from build123d import *

# Parameters (mm, degrees)
SKETCH1_W                                      = 60.6552
SKETCH1_H                                      = 128.4986
BOSS_EXTRUDE1_DEPTH                            = 2.54
CSK_FOR_M3_FLAT_HEAD_MACHINE_SCREW1_AT_2_COUNT = 2
CSK_FOR_M3_FLAT_HEAD_MACHINE_SCREW1_AT_2_PITCH = 75.0062
M3_CLEARANCE_SLOT1_DEPTH                       = 2.54
F_1_4_CLEARANCE_HOLE1_D                        = 7.14248
F_1_4_CLEARANCE_HOLE2_D                        = 6.5278
F_3_8_CLEARANCE_HOLE2_D                        = 10.0838
F_10_CLEARANCE_HOLE1_D                         = 5.6134
CSK_FOR_M2_5_FLAT_HEAD_MACHINE_SCREW1_AT_COUNT = 2
CSK_FOR_M2_5_FLAT_HEAD_MACHINE_SCREW1_AT_PITCH = 25.4
F_11_64_0_17188_DIAMETER_HOLE1_D               = 4.365752
F_6_CLEARANCE_HOLE1_D                          = 4.3053


# Read off the part's stored shape, not the designer's step: M3 Clearance Slot1
with BuildPart() as part:
    # Sketch1 → Boss-Extrude1 (new body)
    with BuildSketch(Plane(origin=(0, 0, 0), x_dir=(1, 0, 0), z_dir=(0, 1, 0))):
        Rectangle(SKETCH1_W, SKETCH1_H)
    extrude(amount=BOSS_EXTRUDE1_DEPTH)

    # Sketch5 → CSK for M3 Flat Head Machine Screw1 (revolve, cut)
    with BuildSketch(Plane(origin=(25.4, 0, -37.5031), x_dir=(0, 0, -1), z_dir=(1, 0, 0))):
        Polygon((0, 0), (0, 2.54), (1.8, 2.54), (1.8, 1.35), (3.15, 0), align=None)
    csk_for_m3_flat_head_machine_screw1 = revolve(axis=Axis((25.4, -6.35, -37.5031), (0, 1, 0)), mode=Mode.SUBTRACT)

    # CSK for M3 Flat Head Machine Screw1 at 2: CSK for M3 Flat Head Machine Screw1 ×2
    with Locations(*[(0, 0, i * CSK_FOR_M3_FLAT_HEAD_MACHINE_SCREW1_AT_2_PITCH) for i in range(1, CSK_FOR_M3_FLAT_HEAD_MACHINE_SCREW1_AT_2_COUNT)]):
        add(csk_for_m3_flat_head_machine_screw1, mode=Mode.SUBTRACT)

    # M3 Clearance Slot1 outline → M3 Clearance Slot1 (cut)
    with BuildSketch(Plane(origin=(0, 0, 0), x_dir=(1, 0, 0), z_dir=(0, 1, 0))):
        with BuildLine():
            ThreePointArc((24.11, -63.0021), (25.86, -61.2521), (24.11, -59.5021))
            Line((24.11, -59.5021), (21.61, -59.5021))
            ThreePointArc((21.61, -59.5021), (19.86, -61.2521), (21.61, -63.0021))
            Line((21.61, -63.0021), (24.11, -63.0021))
        make_face()
        with BuildLine():
            ThreePointArc((24.11, 59.5021), (25.86, 61.2521), (24.11, 63.0021))
            Line((24.11, 63.0021), (21.61, 63.0021))
            ThreePointArc((21.61, 63.0021), (19.86, 61.2521), (21.61, 59.5021))
            Line((21.61, 59.5021), (24.11, 59.5021))
        make_face()
    m3_clearance_slot1 = extrude(amount=M3_CLEARANCE_SLOT1_DEPTH, mode=Mode.SUBTRACT)

    # Mirror1: CSK for M3 Flat Head Machine Screw1, M3 Clearance Slot1 across plane
    add(csk_for_m3_flat_head_machine_screw1.mirror(Plane(origin=(0, 0, 0), x_dir=(0, 0, 1), z_dir=(1, 0, 0))), mode=Mode.SUBTRACT)
    add(m3_clearance_slot1.mirror(Plane(origin=(0, 0, 0), x_dir=(0, 0, 1), z_dir=(1, 0, 0))), mode=Mode.SUBTRACT)

    # Mirror1 copy 1 sketch → Mirror1 copy 1 (revolve, cut)
    with BuildSketch(Plane(origin=(-25.4, 0, 37.5031), x_dir=(0, 0, -1), z_dir=(-1, 0, 0))):
        Polygon((0, 0), (0, -2.54), (1.8, -2.54), (1.8, -1.35), (3.15, 0), align=None)
    revolve(axis=Axis((-25.4, -6.35, 37.5031), (0, -1, 0)), mode=Mode.SUBTRACT)

    # 1/4 Clearance Hole1 (through all)
    with Locations(Plane(origin=(0, 0, 0), x_dir=(-1, 0, 0), z_dir=(0, -1, 0))):
        with Locations((16.3576, 35.0012), (16.3576, 21.301199968), (16.3576, -32.798800036)):
            Hole(F_1_4_CLEARANCE_HOLE1_D / 2)

    # 1/4 Clearance Hole2 (through all)
    with Locations(Plane(origin=(0, 0, 0), x_dir=(-1, 0, 0), z_dir=(0, -1, 0))):
        with Locations((-12.2174, 35.0012), (2.0701, 35.0012), (2.0701, 21.301199968), (-12.2174, 21.301199968), (-12.2174, -17.08879996), (2.0701, -32.798800036)):
            Hole(F_1_4_CLEARANCE_HOLE2_D / 2)

    # 3/8 Clearance Hole2 (through all)
    with Locations(Plane(origin=(0, 0, 0), x_dir=(-1, 0, 0), z_dir=(0, -1, 0))):
        with Locations((9.7536, -17.08879996), (-5.07365, 2.731200024)):
            Hole(F_3_8_CLEARANCE_HOLE2_D / 2)

    # #10 Clearance Hole1 (through all)
    with Locations(Plane(origin=(0, 0, 0), x_dir=(-1, 0, 0), z_dir=(0, -1, 0))):
        with Locations((-12.2174, -32.798800036)):
            Hole(F_10_CLEARANCE_HOLE1_D / 2)

    # Sketch73 → CSK for M2.5 Flat Head Machine Screw1 (revolve, cut)
    with BuildSketch(Plane(origin=(-12.7, 2.54, 49.2633), x_dir=(0, 0, 1), z_dir=(1, 0, 0))):
        Polygon((0, 0), (0, 2.54), (1.45, 2.54), (1.45, 1.3), (2.75, 0), align=None)
    csk_for_m2_5_flat_head_machine_screw1 = revolve(axis=Axis((-12.7, 8.89, 49.2633), (0, -1, 0)), mode=Mode.SUBTRACT)

    # CSK for M2.5 Flat Head Machine Screw1 at: CSK for M2.5 Flat Head Machine Screw1 ×2
    with Locations(*[(i * CSK_FOR_M2_5_FLAT_HEAD_MACHINE_SCREW1_AT_PITCH, 0, 0) for i in range(1, CSK_FOR_M2_5_FLAT_HEAD_MACHINE_SCREW1_AT_COUNT)]):
        add(csk_for_m2_5_flat_head_machine_screw1, mode=Mode.SUBTRACT)

    # 11/64 (0.17188) Diameter Hole1 (through all)
    with Locations(Plane(origin=(0, 0, 0), x_dir=(-1, 0, 0), z_dir=(0, -1, 0))):
        with Locations((11.938, 9.731199994), (11.938, 2.731200024), (11.938, -4.268799946)):
            Hole(F_11_64_0_17188_DIAMETER_HOLE1_D / 2)

    # #6 Clearance Hole1 (through all)
    with Locations(Plane(origin=(0, 2.54, 0), x_dir=(1, 0, 0), z_dir=(0, 1, 0))):
        with Locations((-22.567944323, 48.012104001), (-22.567944323, -48.012104001)):
            f_6_clearance_hole1 = Hole(F_6_CLEARANCE_HOLE1_D / 2)

    # Mirror2: #6 Clearance Hole1 across plane
    add(f_6_clearance_hole1.mirror(Plane(origin=(0, 0, 0), x_dir=(0, 0, 1), z_dir=(1, 0, 0))), mode=Mode.SUBTRACT)


solid = part.part
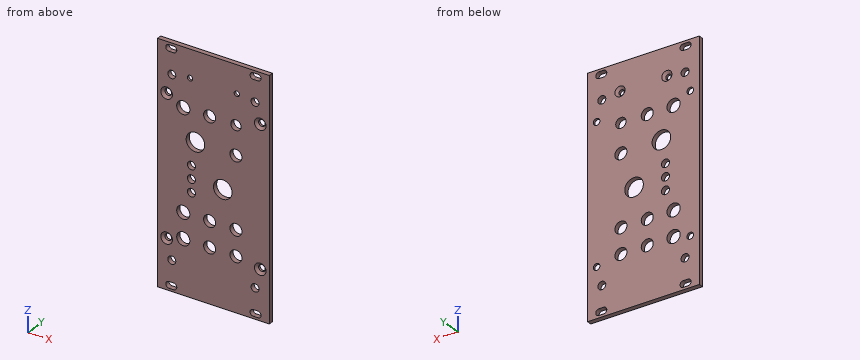
Geometry check sheet. Reference: the model listing, model coordinates, mm. Round coordinates to 2 decimals unless told otherwise and drop trailing zeros. Order: outer loops, then holes, each group sorted by start corner. A loop starts at its lowest first (then second) coordinate and runs counter-clockwise, first axis right, second up. Notation, with made-up numbers: M -32.5,-39.5 L 10.5,-39.5 A21 ccw 10.5,-9.5 Z; hole C 76.25,-2 d9. An arc over 180 degrees is marked long. Answer in a Markdown table with one row per item. Add a question column.
Item 1: Sectioned sample at B-B, the plane z = -20. Enter the section's corners in (x, y).
Item 2: Sectioned sample at A-A, the plane x = 12.7. Enter the section's corners in (y, z), plus the area to 3 significant figures.
Item 3: Depth check by flat-ended pin: pin 1 Ø2.5 at (x, z) = (22.57, 48.01) entering from +Y. Enter the tip coordinate at first touch or a pass-through.
Item 4: Material ranges on L1, parallel to Z at x = -15, y = 0.2; L2, parallel to Z at x = 10.5, y = 1.3; L3, parallel to Z at x = -0.5, y = 2.35, recorded low to high. Write a range as [from, to].
Item 5: Sectioned sample at C-C, the plane y = 0.4. State how many separate pieces and enclosed holes the cut face has, plus the area to 3 significant figures.
Filled in:
| question | item | result |
|---|---|---|
| 1 | outline | M -30.33,0 L -19.68,0 L -19.68,2.54 L -30.33,2.54 Z; M -13.03,0 L -5.06,0 L -5.06,2.54 L -13.03,2.54 Z; M 0.92,0 L 9.22,0 L 9.22,2.54 L 0.92,2.54 Z; M 15.21,0 L 30.33,0 L 30.33,2.54 L 15.21,2.54 Z |
| 2 | outline | M 0,-64.25 L 2.54,-64.25 L 2.54,-38.23 L 0,-38.23 Z; M 0,-31.77 L 2.54,-31.77 L 2.54,-24.53 L 0,-24.53 Z; M 0,-18.07 L 2.54,-18.07 L 2.54,13.86 L 0,13.86 Z; M 0,20.32 L 2.54,20.32 L 2.54,30.03 L 0,30.03 Z; M 0,35.56 L 2.54,35.56 L 2.54,46.51 L 1.24,47.81 L 0,47.81 Z; M 0,50.71 L 1.24,50.71 L 2.54,52.01 L 2.54,64.25 L 0,64.25 Z |
| 2 | area | 254 mm² |
| 3 | pin 1 | passes through |
| 4 | L1 | z = [-64.25, -38.3], [-31.7, -24.6], [-18, 29.5], [36.1, 64.25] |
| 4 | L2 | z = [-64.25, -37.78], [-32.23, -24.08], [-18.53, 14.31], [19.86, 30.58], [35.02, 64.25] |
| 4 | L3 | z = [-64.25, -37.86], [-32.14, -24.16], [-18.44, 29.94], [35.66, 64.25] |
| 5 | separate pieces | 1 |
| 5 | enclosed holes | 29 |
| 5 | area | 7,000 mm² |
